```python
from build123d import *

# Parameters (mm, degrees)
SKETCH1_W           = 50.8
SKETCH1_H           = 25.4
SKETCH1_W_2         = 44.45
SKETCH1_H_2         = 19.05
EXTRUDE_THIN1_DEPTH = 19.05
SKETCH2_R           = 2.4892
CUT_EXTRUDE1_DEPTH  = 26.4


with BuildPart() as part:
    # Sketch1 → Extrude-Thin1 (new body, symmetric)
    with BuildSketch(Plane.XY):
        with Locations((25.4, 12.7)):
            Rectangle(SKETCH1_W, SKETCH1_H)
        with Locations((25.4, 12.7)):
            Rectangle(SKETCH1_W_2, SKETCH1_H_2, mode=Mode.SUBTRACT)
    extrude(amount=EXTRUDE_THIN1_DEPTH, both=True)

    # Sketch2 → Cut-Extrude1 (cut, through all)
    with BuildSketch(Plane(origin=(0, 25.4, 0), x_dir=(1, 0, 0), z_dir=(0, 1, 0))):
        with Locations((38.1, 6.35)):
            Circle(SKETCH2_R)
        with Locations((38.1, -6.35)):
            Circle(SKETCH2_R)
        with Locations((12.7, -6.35)):
            Circle(SKETCH2_R)
        with Locations((12.7, 6.35)):
            Circle(SKETCH2_R)
    extrude(amount=-CUT_EXTRUDE1_DEPTH, mode=Mode.SUBTRACT)


solid = part.part
```
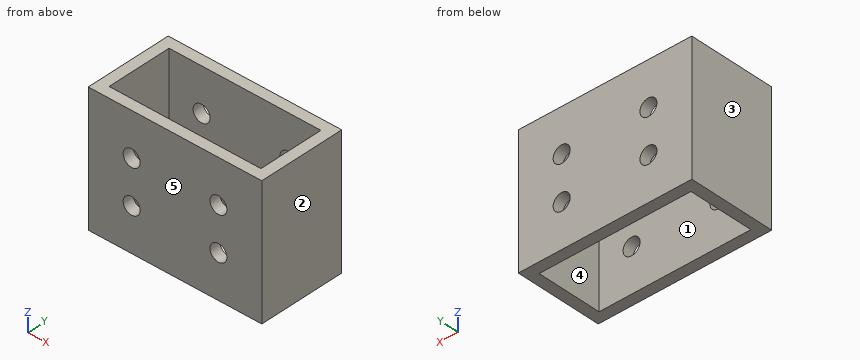
For this review, take the finished solid that the model builds, in its own axes (mm). Face numbers are marked on the shaded views. A direction names the side the tool comes from. Round coordinates to 2 decimals unless told otherwise and drop trailing zeros. Write each loop counter-clockwise with the first axis right and the second up, starting at its lowest first coordinate (ties: lowest second). Pieces come first, ordered by that corner, then holes. Notation, with made-up numbers: (-18.75, 33) - (4.25, 33) arc R27 ccw to (4.25, 67) - close; hole circle Ø10 at (-1, 9). An arc over 180 degrees is marked (long way). Use CSV: the item, a comma, the result in double quotes.
1) For the marked faces 1 and 2, list the 3-axis set-ups (+Z, -Z, +X, -X, +Y, -Y) from which the entire face can be reached by the end or side of a thin tool; tool diameter is ignored.
Conclusion:
face 1,"+Z, -Z"
face 2,"+Z, -Z, +X, +Y, -Y"
2) Wall thickness on line 1 along X through (y, z) = (23.25, 6.35); line 2 along Z through (x, y) = (38.1, 0.8); line 3 along Y through (x, z) = (4, -11) (3 decimals): over which ranges is each line inside the solid? List them lowest first. Write a range as from..to.
Conclusion:
line 1,"x = 0..10.21, 15.19..35.61, 40.59..50.8"
line 2,"z = -19.05..-8.84, -3.86..3.86, 8.84..19.05"
line 3,"y = 0..3.175, 22.225..25.4"
3) Add section D-D on z = -13.5. Write out the cut boundary in (x, y) (3 decimals), and give its area (3 significant figures).
Conclusion:
outline,"(0, 0) - (50.8, 0) - (50.8, 25.4) - (0, 25.4) - close; hole (3.175, 3.175) - (47.625, 3.175) - (47.625, 22.225) - (3.175, 22.225) - close"
area,"444 mm^2"
4) Add section A-A on x = 4.5. Write out the cut boundary in (y, z) (3 decimals), and give its area (3 significant figures).
Conclusion:
outline,"(0, -19.05) - (3.175, -19.05) - (3.175, 19.05) - (0, 19.05) - close; (22.225, -19.05) - (25.4, -19.05) - (25.4, 19.05) - (22.225, 19.05) - close"
area,"242 mm^2"
5) Add section C-C on x = 38.1. Write out the cut boundary in (y, z) (3 decimals).
Conclusion:
outline,"(0, -19.05) - (3.175, -19.05) - (3.175, -8.839) - (0, -8.839) - close; (0, -3.861) - (3.175, -3.861) - (3.175, 3.861) - (0, 3.861) - close; (0, 8.839) - (3.175, 8.839) - (3.175, 19.05) - (0, 19.05) - close; (22.225, -19.05) - (25.4, -19.05) - (25.4, -8.839) - (22.225, -8.839) - close; (22.225, -3.861) - (25.4, -3.861) - (25.4, 3.861) - (22.225, 3.861) - close; (22.225, 8.839) - (25.4, 8.839) - (25.4, 19.05) - (22.225, 19.05) - close"
6) The part is to be moulded in two halves that separate along Y. For the marked faces 3, 4 and 5, say which applies: pulls with the +Y half, pulls with the -Y half, needs draft (parallel to the pull), parting line crosses it, or undercut.
Conclusion:
face 3,"needs draft"
face 4,"undercut"
face 5,"pulls with the -Y half"
7) Clearance check with a flat-ended pin moving along its axis: pin 1 Ø4 at (x, z) = (38.1, -6.35) entering from -Y. State where the tip first meets the part, or that it passes through.
Conclusion:
pin 1,"passes through"
8) Add section B-B on z = -6.35. Write out the cut boundary in (x, y) (3 decimals), and give its area (3 significant figures).
Conclusion:
outline,"(0, 0) - (10.211, 0) - (10.211, 3.175) - (3.175, 3.175) - (3.175, 22.225) - (10.211, 22.225) - (10.211, 25.4) - (0, 25.4) - close; (15.189, 0) - (35.611, 0) - (35.611, 3.175) - (15.189, 3.175) - close; (15.189, 22.225) - (35.611, 22.225) - (35.611, 25.4) - (15.189, 25.4) - close; (40.589, 0) - (50.8, 0) - (50.8, 25.4) - (40.589, 25.4) - (40.589, 22.225) - (47.625, 22.225) - (47.625, 3.175) - (40.589, 3.175) - close"
area,"380 mm^2"
